Source: CAD feature listing. Evaluate the final solid. Frame: model axes, mm. A direction names the side the tool comes from. Round coordinates to 2 decimals unless told otherwise and drop trailing zeros. Order: outer loops, then holes, each group sorted by start corner. A loop starts at its lowest first (then second) coordinate and runs counter-clockwise, first axis right, second up. Notation, with made-up numbers: (-2.75, -34.5) -> (38.25, -34.5) arc R24 cw to (38.25, -24.5) -> close; hole circle Ø11 at (45, -1). An arc over 180 degrees is marked (long way). One line per item, written item: value. Start each with the question number.
1) Section D-D (z = 7.75). Return the cut outline in (x, y), and give its area (3 significant figures).
2) Mould query, pull axis X, two halves, no side actions, for faces 4 (the face through (-2.2, -1.1, 23.5)), 5 (the face through (5.07, 0.67, 22.23)), 6 (the face through (1, -1, 21.1)). Classes: pulls with the +X half, pulls with the -X half, needs draft (parallel to the pull), parting line crosses it, or undercut.
3) Pin query (flat end, axial travel): P1, Ø5, axis at x = 3.5, z = 22, coming from the +Y side; P2, Ø1, axis at y = -1.5, z = 14, coming from the +X side; P3, Ø3, axis at x = 0, y = 2.11, coming from the +Z side. Return the tip coordinate at first contact, or that it passes through.
4) Reachability of faces 1 (the face through (1, 1, 26.1)), 2 (the face through (-0.7, -4.2, 22.3)), 3 (the face through (-7.493, 0.33, 7.888)) from +Z, -Z, +X, -X, +Y, -Y: full face, straight path, thin tool, end or side. Return the list, or none.
5) Section A-A (x = 4.75). Return the cut outline in (y, z).
6) Section B-B (y = 3). Return the cut outline in (x, z), and give its area (3 significant figures).
7) Section C-C (z = 11.5). Return the cut outline in (x, y), and give its area (3 significant figures).
8) Ray query, L1, parallel to Z at x = 5, y = 0.5; L2, parallel to Y at x = 0, z = 17; L3, parallel to Z at x = 5, y = -1.75. Return the intervals inside material, ascending.
```python
from build123d import *

# Parameters (mm, degrees)
SKETCH1_R                                           = 7.5
BOSS_EXTRUDE1_DEPTH                                 = 16
SKETCH2_R                                           = 3
BOSS_EXTRUDE2_DEPTH                                 = 5
SKETCH3_R                                           = 5.1125
BOSS_EXTRUDE3_DEPTH                                 = 2.5
SKETCH5_R                                           = 3
BOSS_EXTRUDE4_DEPTH                                 = 5
CBORE_FOR_M2_HEX_SOCKET_HEAD_CAP_SCREW1_D           = 2.4
CBORE_FOR_M2_HEX_SOCKET_HEAD_CAP_SCREW1_DEPTH       = 7.5
CBORE_FOR_M2_HEX_SOCKET_HEAD_CAP_SCREW1_CBORE_D     = 4.4
CBORE_FOR_M2_HEX_SOCKET_HEAD_CAP_SCREW1_CBORE_DEPTH = 2.4


with BuildPart() as part:
    # Sketch1 → Boss-Extrude1 (new body)
    with BuildSketch(Plane.XY):
        Circle(SKETCH1_R)
    extrude(amount=BOSS_EXTRUDE1_DEPTH)

    # Sketch2 → Boss-Extrude2 (add)
    with BuildSketch(Plane.XY.offset(16)):
        with Locations((0, -2.1125)):
            Circle(SKETCH2_R)
    extrude(amount=BOSS_EXTRUDE2_DEPTH)

    # Sketch3 → Boss-Extrude3 (add)
    with BuildSketch(Plane.XY.offset(21)):
        with Locations(Location((0, 0, 0), (0, 0, 270))):
            Circle(SKETCH3_R)
    extrude(amount=BOSS_EXTRUDE3_DEPTH)

    # Sketch5 → Boss-Extrude4 (add)
    with BuildSketch(Plane.XY.offset(23.5)):
        with Locations(Location((0, 2.1125, 0), (0, 0, 90))):
            Circle(SKETCH5_R)
    extrude(amount=BOSS_EXTRUDE4_DEPTH)

    # CBORE for M2 Hex Socket Head Cap Screw1
    with Locations(Plane.XY.offset(28.5)):
        with Locations((0, 2.1125)):
            CounterBoreHole(CBORE_FOR_M2_HEX_SOCKET_HEAD_CAP_SCREW1_D / 2, CBORE_FOR_M2_HEX_SOCKET_HEAD_CAP_SCREW1_CBORE_D / 2, CBORE_FOR_M2_HEX_SOCKET_HEAD_CAP_SCREW1_CBORE_DEPTH, depth=CBORE_FOR_M2_HEX_SOCKET_HEAD_CAP_SCREW1_DEPTH)

    # Sketch10 → CBORE for M2 Hex Socket Head Cap Screw2 (revolve, cut)
    with BuildSketch(Plane(origin=(0, -2.1125, 23.5), x_dir=(0, -1, 0), z_dir=(1, 0, 0))):
        Polygon((0, 0), (0, 14.721032743), (1.2, 14), (1.2, 2.4), (2.2, 2.4), (2.2, 0), align=None)
    revolve(axis=Axis((0, -2.1125, 29.85), (0, 0, -1)), mode=Mode.SUBTRACT)


solid = part.part
```
Findings:
1. outline: circle Ø15 at (0, 0)
1. area: 177 mm2
2. face 4: needs draft
2. face 5: parting line crosses it
2. face 6: undercut
3. P1: y = 5.01
3. P2: x = 7.43
3. P3: z = 26.1
4. face 1: +Z
4. face 2: none
4. face 3: +Z, -Z
5. outline: (-5.8, 0) -> (5.8, 0) -> (5.8, 16) -> (-5.8, 16) -> close; (-1.89, 21) -> (1.89, 21) -> (1.89, 23.5) -> (-1.89, 23.5) -> close
6. outline: (-6.87, 0) -> (6.87, 0) -> (6.87, 16) -> (-6.87, 16) -> close; (-4.14, 21) -> (-0.81, 21) -> (-0.81, 26.1) -> (-2.01, 26.1) -> (-2.01, 28.5) -> (-2.87, 28.5) -> (-2.87, 23.5) -> (-4.14, 23.5) -> close; (0.81, 21) -> (4.14, 21) -> (4.14, 23.5) -> (2.87, 23.5) -> (2.87, 28.5) -> (2.01, 28.5) -> (2.01, 26.1) -> (0.81, 26.1) -> close
6. area: 251 mm2
7. outline: circle Ø15 at (0, 0); hole circle Ø2.4 at (0, -2.11)
7. area: 172 mm2
8. L1: 0 to 16, 21 to 23.5
8. L2: -5.11 to -3.31, -0.91 to 0.89
8. L3: 0 to 16
